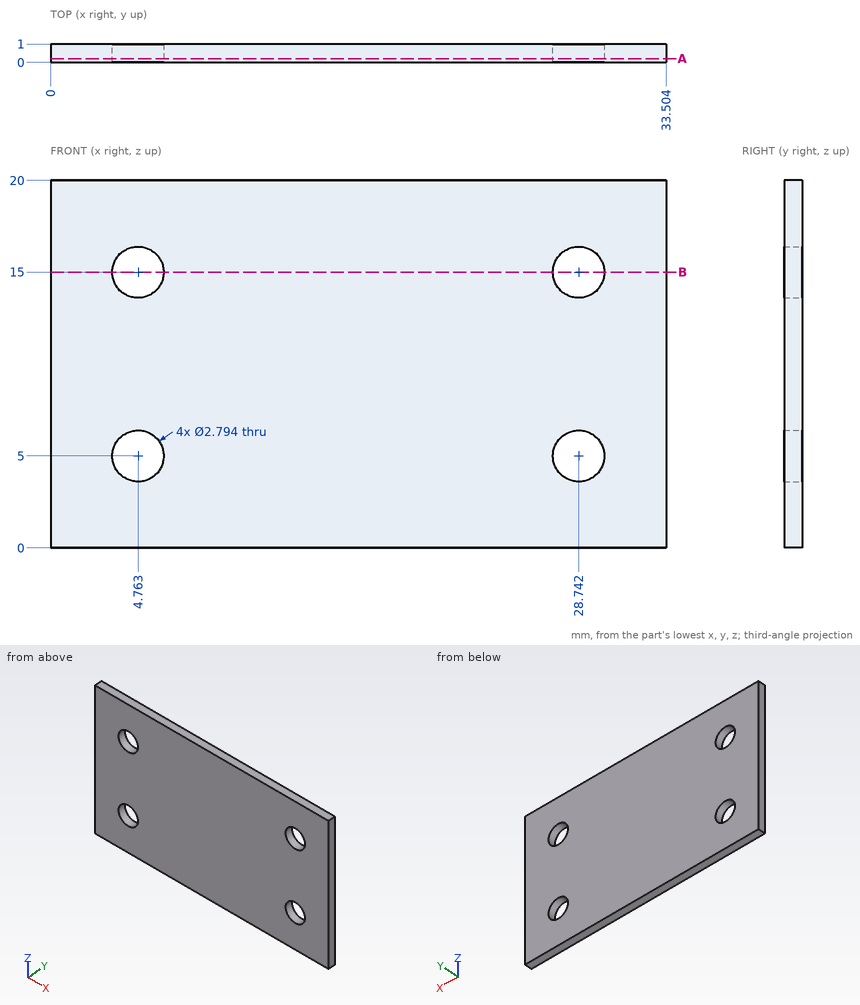
Study the drawing (mm; zero at the part's minimum x, y, z) and answer. Give positions to 0.01 mm unless a question says otherwise; leave off trailing zeros. Write each loop counter-clockwise with the first axis right and the second up, starting at its lowest first coordinate (ties: lowest second). Pieces come first, ordered by that corner, then holes. Notation, with made-up numbers: (-11, 25.25) - (26, 25.25) arc R16 cw to (26, 36.25) - close; hole circle Ø2 at (-27.75, 1.25). An arc over 180 degrees is marked (long way). Use CSV: the item, a comma, the result in double quotes. Start each with the question number.
(1) Find section A-A (y = 0.2). Give the vertices of the cut face in (x, z) (1 decimal).
(2) Given P1, Ø2, axis at x = 28.74, z = 5, coming from the +Y side; P2, Ø1.5, axis at x = 7.5, z = 12.5, coming from the -Y side, each flat-ended and moving along its own axis, determine where each tip first touches the part or whether it passes through.
(3) Find section B-B (z = 15). Give the vertices of the cut face in (x, y) (1 decimal).
(4) Consider line 1 along X through (y, z) = (0.55, 5) (1 decimal); line 2 along Z through (x, y) = (30, 0.6) (1 decimal); line 3 along Z through (x, y) = (4, 0.1). Determine where each line is inside the solid, lowest interval first.
Findings below:
1,outline,"(0, 0) - (33.5, 0) - (33.5, 20) - (0, 20) - close; hole circle Ø2.8 at (4.8, 5); hole circle Ø2.8 at (4.8, 15); hole circle Ø2.8 at (28.7, 5); hole circle Ø2.8 at (28.7, 15)"
2,P1,"through"
2,P2,"y = 0"
3,outline,"(0, 0) - (3.4, 0) - (3.4, 1) - (0, 1) - close; (6.2, 0) - (27.3, 0) - (27.3, 1) - (6.2, 1) - close; (30.1, 0) - (33.5, 0) - (33.5, 1) - (30.1, 1) - close"
4,line 1,"0 to 3.4, 6.2 to 27.3, 30.1 to 33.5"
4,line 2,"0 to 4.4, 5.6 to 14.4, 15.6 to 20"
4,line 3,"0 to 3.83, 6.17 to 13.83, 16.17 to 20"
